Build history of the part. All positions in model axes, mm. Face numbers are marked on the shaded views. A direction names the side the tool comes from. Round coordinates to 2 decimals unless told otherwise and drop trailing zeros. Order: outer loops, then holes, each group sorted by start corner. A loop starts at its lowest first (then second) coordinate and runs counter-clockwise, first axis right, second up. Notation, with made-up numbers: (-7.5, -0.5) -> (24.5, -0.5) arc R11 ccw to (24.5, 18.5) -> close; hole circle Ø7 at (-17, -10). An arc over 180 degrees is marked (long way). Use a Markdown table: item, result. Add a question column.
Item 1: Pin check, flat tips, straight feed: pin 1 (11.5 mm diameter, centred on x = 31.5, y = -8, fed in from -Z); pin 2 (6 mm diameter, centred on x = -9, y = -16.5, fed in from -Z); pin 3 (3 mm diameter, centred on x = 20.5, y = -13, fed in from -Z). Stop position of each tip, or through.
Item 2: Slice it at C-C, the plane y = -11.75. Give the cut face in (x, z), plus the area to 3 significant figures.
Item 3: Probe L1, parallel to X at y = -18, z = 27; L2, parallel to Z at x = -38, y = -15.5; L3, parallel to Z at x = -25.5, y = -17.75. List the from-to ranges inside material, lowest first.
Item 4: Slice it at A-A, the plane x = 0. Give the cut face in (y, z).
Item 5: Slice it at D-D, the plane y = -4.25. State how many separate pieces and enclosed holes the cut face has, plus the area to 3 significant figures.
Item 6: Slice it at B-B, the plane z = 0. Give the cut face in (x, y).
Item 7: 3-axis set-ups, long thin cutter, end or side, ignore diameter. For the marked faces 5 and 6: which of +Z, -Z, +X, -X, +Y, -Y reach the whole face in a straight line?
Item 8: Two-plate mould, pull along Z, no slides. Class the marked faces 1, 2, 3 and 4: released by +Z, released by -Z, zero draft, split by the parting line, or undercut.
from build123d import *

# Parameters (mm, degrees)
SKETCH1_R             = 60
BOSS_EXTRUDE1_DEPTH   = 20
BOSS_EXTRUDE1_DRAFT   = -40
CUT_EXTRUDE1_DEPTH    = 25
F_3_0MM_DOWEL_HOLE1_D = 3
FILLET1_R             = 8
SKETCH13_R            = 2.5
CUT_EXTRUDE5_DEPTH    = 10


with BuildPart() as part:
    # Sketch1 → Boss-Extrude1 (with draft: the straight prism first)
    with BuildSketch(Plane(origin=(0, 0, 0), x_dir=(1, 0, 0), z_dir=(0, 1, 0))):
        Circle(SKETCH1_R)
    extrude(amount=-BOSS_EXTRUDE1_DEPTH)
    # Boss-Extrude1: the draft: its side faces are tilted about the plane it starts from
    boss_extrude1_sides = [part.faces().sort_by_distance(p)[0] for p in [
        (-60, -10, 0),
    ]]
    draft(boss_extrude1_sides, Plane(origin=(0, 0, 0), x_dir=(1, 0, 0), z_dir=(0, 1, 0)), BOSS_EXTRUDE1_DRAFT)

    # Sketch5 → Cut-Extrude1 (cut)
    with BuildSketch(Plane.XZ.offset(20)):
        with BuildLine():
            Line((-20, 20), (-20, 38.311827959))
            ThreePointArc((-20, 38.311827959), (-30.559746085, 30.559746085), (-38.311827959, 20))
            Line((-38.311827959, 20), (-20, 20))
        make_face()
        with BuildLine():
            ThreePointArc((38.311827959, 20), (30.559746085, 30.559746085), (20, 38.311827959))
            Line((20, 38.311827959), (20, 20))
            Line((20, 20), (38.311827959, 20))
        make_face()
        with BuildLine():
            Line((-20, -20), (-38.311827959, -20))
            ThreePointArc((-38.311827959, -20), (-30.559746085, -30.559746085), (-20, -38.311827959))
            Line((-20, -38.311827959), (-20, -20))
        make_face()
        with BuildLine():
            ThreePointArc((20, -38.311827959), (30.559746085, -30.559746085), (38.311827959, -20))
            Line((38.311827959, -20), (20, -20))
            Line((20, -20), (20, -38.311827959))
        make_face()
    extrude(amount=-CUT_EXTRUDE1_DEPTH, mode=Mode.SUBTRACT)

    # Ø3.0mm Dowel Hole1 (through all)
    with Locations(Plane(origin=(0, -20, 0), x_dir=(-1, 0, 0), z_dir=(0, -1, 0))):
        with Locations((0, -34.64), (-29.999119987, 17.32), (29.999119987, 17.32)):
            Hole(F_3_0MM_DOWEL_HOLE1_D / 2)

    # Fillet1
    fillet1_edges = [part.edges().sort_by_distance(p)[0] for p in [
        (-20, -10, -20),
        (20, -10, -20),
        (20, -10, 20),
        (-20, -10, 20),
    ]]
    fillet(fillet1_edges, radius=FILLET1_R)

    # Sketch13 → Cut-Extrude5 (cut)
    with BuildSketch(Plane(origin=(0, 0, 0), x_dir=(1, 0, 0), z_dir=(0, 1, 0))):
        with Locations(Location((0, 30, 0), (0, 0, 270))):
            Circle(SKETCH13_R)
        with Locations(Location((30, 0, 0), (0, 0, 270))):
            Circle(SKETCH13_R)
        with Locations(Location((0, -30, 0), (0, 0, 270))):
            Circle(SKETCH13_R)
        with Locations(Location((-30, 0, 0), (0, 0, 270))):
            Circle(SKETCH13_R)
    extrude(amount=-CUT_EXTRUDE5_DEPTH, mode=Mode.SUBTRACT)


solid = part.part
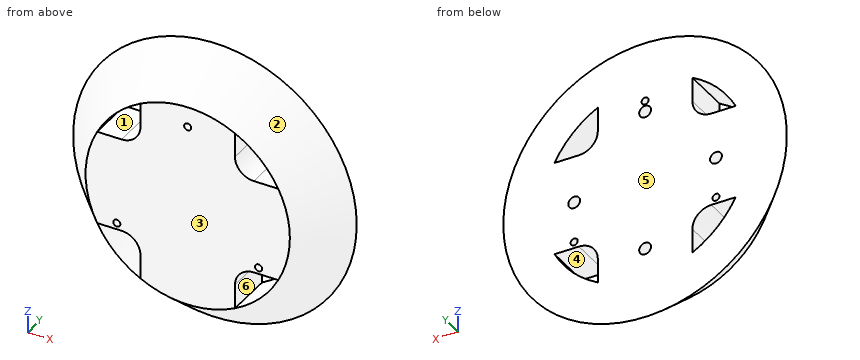
Check sheet entries:
| question | item | result |
|---|---|---|
| 1 | pin 1 | z = -49.83 |
| 1 | pin 2 | z = -47.89 |
| 1 | pin 3 | z = -46.14 |
| 2 | outline | circle Ø100.28 at (0, 0); hole (-38.31, -20) arc R43.22 ccw to (-20, -38.31) -> (-20, -28) arc R8 ccw to (-28, -20) -> close; hole (-38.31, 20) -> (-28, 20) arc R8 ccw to (-20, 28) -> (-20, 38.31) arc R43.22 ccw to start; hole circle Ø3 at (-30, -17.32); hole circle Ø3 at (0, 34.64); hole (20, -38.31) arc R43.22 ccw to (38.31, -20) -> (28, -20) arc R8 ccw to (20, -28) -> close; hole (20, 28) arc R8 ccw to (28, 20) -> (38.31, 20) arc R43.22 ccw to (20, 38.31) -> close; hole circle Ø3 at (30, -17.32) |
| 2 | area | 7,120 mm2 |
| 3 | L1 | -35.87 to -33.75, -20.06 to 20.06, 33.75 to 35.87 |
| 3 | L2 | -27.65 to -20.59, -20 to 20, 20.59 to 27.65 |
| 3 | L3 | -37.21 to -34.89, -20.4 to 20.4, 34.89 to 37.21 |
| 4 | outline | (-20, -43.22) -> (0, -60) -> (0, -32.5) -> (-10, -32.5) -> (-10, -27.5) -> (0, -27.5) -> (0, 27.5) -> (-10, 27.5) -> (-10, 32.5) -> (0, 32.5) -> (0, 33.14) -> (-20, 33.14) -> close; (-20, 36.14) -> (0, 36.14) -> (0, 60) -> (-20, 43.22) -> close |
| 5 | separate pieces | 1 |
| 5 | enclosed holes | 11 |
| 5 | area | 9,150 mm2 |
| 6 | outline | (-60, 0) -> (-43.22, -20) -> (43.22, -20) -> (60, 0) -> (32.5, 0) -> (32.5, -10) -> (27.5, -10) -> (27.5, 0) -> (-27.5, 0) -> (-27.5, -10) -> (-32.5, -10) -> (-32.5, 0) -> close |
| 7 | face 5 | +Z, -Z, +X, -X, +Y |
| 7 | face 6 | +Y, -Y |
| 8 | face 1 | undercut |
| 8 | face 2 | split by the parting line |
| 8 | face 3 | zero draft |
| 8 | face 4 | undercut |
